Work out the finished part from the listing and answer in its coordinate system (mm). Face numbers are marked on the shaded views. Coordinates: 2 decimals unless noted, no trailing zeros. Write each loop counter-clockwise with the first axis right and the second up, starting at its lowest first coordinate (ties: lowest second). Pieces come first, ordered by that corner, then holes. Notation, with made-up numbers: M 11,22 L 27,22 A35 ccw 27,59 Z; hole C 87,-32 d1. An arc over 180 degrees is marked long. Answer as CSV lines item,"result". Start each with the question number.
(1) A cutting plane is placed at A-A on x = 9. Give the vertices of the cut face in (y, z).
(2) Find the intervals of material crossed by L1, parallel to Z at x = 9, y = 1.35; L2, parallel to X at y = 1.6, z = -13.5; L3, parallel to X at y = 1.65, z = -18.75, in increasing order. Write a range as [from, to].
(3) A cutting plane is placed at C-C on x = 6.5. Give the vertices of the cut face in (y, z).
(4) The mould has two halves that part along X. Classify the marked faces 1, 2, 3 and 4: released by +X, released by -X, zero draft, split by the parting line, or undercut.
(5) A cutting plane is placed at B-B on z = -6.5. Give the vertices of the cut face in (x, y).
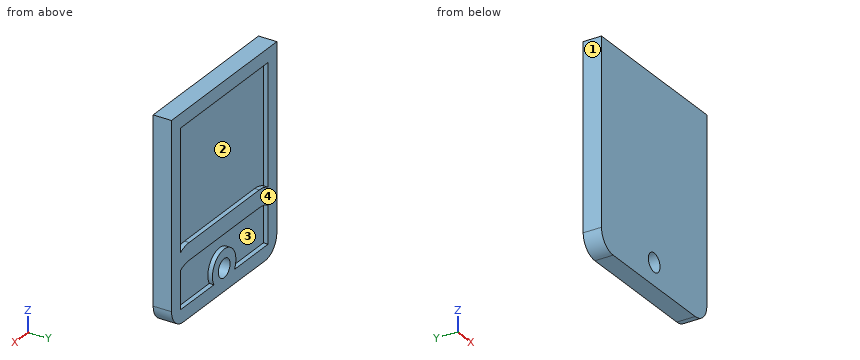
Autodesk Inventor part; units mm, degrees
ref_plane "YZ Plane" through (0, 0, 0) normal (1, 0, 0) x (0, 1, 0)
ref_plane "XZ Plane" through (0, 0, 0) normal (0, 1, 0) x (-1, 0, 0)
ref_plane "XY Plane" through (0, 0, 0) normal (0, 0, 1) x (1, 0, 0)
sketch "Sketch1" plane through (0, 0, 0) normal (0, 1, 0) x (-1, 0, 0)
  line L0 (0, 0) -> (-18, 0)
  line L1 (-18, 0) -> (-18, -22)
  line L2 (-18, -22) -> (0, -22)
  line L3 (0, -22) -> (0, 0)
  line L4 (-1.5, -20.5) -> (2.5, -20.5) construction
  circle A0 centre (-9, -19.8358) radius 1.5
  line L5 (-1, -20.5) -> (-7.6551, -20.5)
  line L6 (-1, -20.5) -> (-1, -1.5)
  line L7 (-1, -1.5) -> (-1, -1)
  line L8 (-1, -1) -> (-17, -1)
  line L9 (-17, -1) -> (-17, -20.5)
  line L10 (-1, -1) -> (-17, -1)
  line L11 (-17, -1) -> (-17, -20.5)
  line L12 (-1, -20.5) -> (-1, -1)
  line L13 (-10.3449, -20.5) -> (-17, -20.5)
  point P0 (0, 0)
  point P1 (-15.5, -20.5)
  dimension "d0" = 18
  dimension "d1" = 22
  dimension "d2" = 3
  dimension "d3" = 0.5
  dimension "d4" = 16
extrude "Extrusion1" add sketch "Sketch1" along normal blind 2 contours L3 L2 L1 L0 | A0 L13 L9 L8 L7 L6 L5
sketch "Sketch8" plane through (0, 2, 0) normal (0, 1, 0) x (1, 0, 0)
  circle A0 centre (9, 19.8358) radius 1.5
  circle A1 centre (9, 19.8358) radius 1.5
  line L0 (0, 0) -> (18, 0)
  line L1 (18, 0) -> (18, 22)
  line L2 (18, 22) -> (0, 22)
  line L3 (0, 22) -> (0, 0)
extrude "Extrusion5" add sketch "Sketch8" against normal blind 2 contours A0
sketch "Sketch9" plane through (0, 2, 0) normal (0, 1, 0) x (1, 0, 0)
  line L0 (0, 0) -> (18, 0)
  line L1 (18, 0) -> (18, 22)
  line L2 (18, 22) -> (0, 22)
  line L3 (0, 22) -> (0, 0)
  line L4 (18, 22) -> (18, 17.1361)
  line L5 (15, 16) -> (3, 16)
  line L6 (0, 17.1361) -> (0, 22)
  arc A0 (0, 19) -> (3, 16) centre (3, 19) ccw
  arc A1 (15, 16) -> (18, 19) centre (15, 19) ccw
  line L7 (15, 16) -> (3, 16)
  arc A2 (0, 19) -> (3, 16) centre (3, 19) ccw
  arc A3 (15, 16) -> (18, 19) centre (15, 19) ccw
  line L8 (15, 14.1361) -> (3, 14.1361)
  arc A4 (0, 17.1361) -> (3, 14.1361) centre (3, 17.1361) ccw
  arc A5 (15, 14.1361) -> (18, 17.1361) centre (15, 17.1361) ccw
  line L9 (15, 14.1361) -> (3, 14.1361)
  arc A6 (0, 17.1361) -> (3, 14.1361) centre (3, 17.1361) ccw
  arc A7 (15, 14.1361) -> (18, 17.1361) centre (15, 17.1361) ccw
  circle A8 centre (9, 19.568) radius 2
  dimension "d19" = 4
extrude "Extrusion6" cut sketch "Sketch9" against normal blind 0.5 contours L3 A4 L8 A5 L1 L0 | L3 L2 L1 A1 L5 A0
sketch "Sketch11" plane through (0, 0, 0) normal (0, -1, 0) x (1, 0, 0)
  line L0 (1.5, -20.5) -> (16.5, -20.5)
  line L1 (16.5, -20.5) -> (16.5, -1.5)
  line L2 (18, -17.1361) -> (18, 0)
  line L3 (0, -22) -> (18, -22)
  line L4 (0, -22) -> (18, -22)
  line L5 (18, -22) -> (18, 0)
  line L6 (16.5, -1.5) -> (1.5, -1.5)
  line L7 (0, -19) -> (0, -22)
  line L8 (1.5, -1.5) -> (1.5, -20.5)
  line L9 (0, 0) -> (0, -22)
  line L10 (0, 0) -> (0, -17.1361)
  line L11 (0, 0) -> (0, -17.1361)
  line L12 (18, -22) -> (18, -19)
  line L13 (18, 0) -> (0, 0)
  line L14 (18, 0) -> (0, 0)
  line L15 (0, 0) -> (18, 0)
  line L16 (18, 0) -> (18, -22)
  line L17 (18, -22) -> (0, -22)
  line L18 (0, -22) -> (0, 0)
  line L19 (16.5, -1.5) -> (1.5, -1.5)
  line L20 (1.5, -1.5) -> (1.5, -20.5)
  line L21 (1.5, -20.5) -> (16.5, -20.5)
  line L22 (16.5, -20.5) -> (16.5, -1.5)
extrude "Extrusion7" add sketch "Sketch11" against normal blind 2
sketch "Sketch12" plane through (0, 2, 0) normal (0, 1, 0) x (1, 0, 0)
  arc A0 (7.2304, 20.5) -> (10.7696, 20.5) centre (9, 19.568) ccw
  circle A1 centre (9, 19.568) radius 1
  point P0 (0, 0)
  dimension "d28" = 2
extrude "Extrusion8" cut sketch "Sketch12" against normal blind 2
fillet "Fillet1" radius 2 2 edges at (0, 1, -22) (18, 1, -22)
properties part number "bolsillop2"
Here are the results:
1,outline,"M 0,-22 L 2,-22 L 2,-20.57 L 0,-20.57 Z; M 0,-18.57 L 2,-18.57 L 2,-17.57 L 1.5,-17.57 L 1.5,-16 L 2,-16 L 2,-14.14 L 1.5,-14.14 L 1.5,-1.5 L 2,-1.5 L 2,0 L 0,0 Z"
2,L1,"z = [-22, -20.57], [-18.57, 0]"
2,L2,"x = [0, 1.5], [16.5, 18]"
2,L3,"x = [0, 1.5], [7.17, 8.42], [9.58, 10.83], [16.5, 18]"
3,outline,"M 0,-22 L 2,-22 L 2,-20.5 L 1.5,-20.5 L 1.5,-16 L 2,-16 L 2,-14.14 L 1.5,-14.14 L 1.5,-1.5 L 2,-1.5 L 2,0 L 0,0 Z"
4,face 1,"released by -X"
4,face 2,"undercut"
4,face 3,"undercut"
4,face 4,"zero draft"
5,outline,"M 0,0 L 18,0 L 18,2 L 16.5,2 L 16.5,1.5 L 1.5,1.5 L 1.5,2 L 0,2 Z"
